Design review of the part built by this model. Coordinates are the model's own, in mm. A direction names the side the tool comes from. Round coordinates to 2 decimals unless told otherwise and drop trailing zeros. Order: outer loops, then holes, each group sorted by start corner. A loop starts at its lowest first (then second) coordinate and runs counter-clockwise, first axis right, second up.
from build123d import *

# Parameters (mm, degrees)
CROQUIS1_R              = 21.4
CROQUIS1_R_2            = 18.65
SALIENTE_EXTRUIR1_DEPTH = 26.4
CROQUIS2_R              = 18.65
SALIENTE_EXTRUIR2_DEPTH = 3
SALIENTE_EXTRUIR3_START = -4
CROQUIS3_R              = 28.5
CROQUIS3_R_2            = 21.4
SALIENTE_EXTRUIR3_DEPTH = 4
CROQUIS4_R              = 6.15
CROQUIS4_R_2            = 1.65
CORTAR_EXTRUIR1_DEPTH   = 3
CROQUIS6_R              = 2
CORTAR_EXTRUIR2_DEPTH   = 49.181531732
CROQUIS7_R              = 21.4
CROQUIS7_R_2            = 20
CORTAR_EXTRUIR3_DEPTH   = 22.4
REDONDEO1_R             = 1


with BuildPart() as part:
    # Croquis1 → Saliente-Extruir1 (new body)
    with BuildSketch(Plane.XY):
        Circle(CROQUIS1_R)
        Circle(CROQUIS1_R_2, mode=Mode.SUBTRACT)
    extrude(amount=SALIENTE_EXTRUIR1_DEPTH)

    # Croquis2 → Saliente-Extruir2 (add)
    with BuildSketch(Plane(origin=(0, 0, 0), x_dir=(-1, 0, 0), z_dir=(0, 0, -1))):
        Circle(CROQUIS2_R)
    extrude(amount=-SALIENTE_EXTRUIR2_DEPTH)

    # Croquis3 → Saliente-Extruir3 (add)
    with BuildSketch(Plane.XY.offset(26.4).offset(SALIENTE_EXTRUIR3_START)):
        Circle(CROQUIS3_R)
        Circle(CROQUIS3_R_2, mode=Mode.SUBTRACT)
    extrude(amount=SALIENTE_EXTRUIR3_DEPTH)

    # Croquis4 → Cortar-Extruir1 (cut)
    with BuildSketch(Plane(origin=(0, 0, 0), x_dir=(-1, 0, 0), z_dir=(0, 0, -1))):
        with Locations((0, -7)):
            Circle(CROQUIS4_R)
        with Locations((-15.497639275, 0.2705123)):
            Circle(CROQUIS4_R_2)
        with Locations((-7.514549114, 13.556605461)):
            Circle(CROQUIS4_R_2)
        with Locations((7.983090161, 13.286093161)):
            Circle(CROQUIS4_R_2)
        with Locations((15.497639275, -0.2705123)):
            Circle(CROQUIS4_R_2)
        with Locations((7.514549114, -13.556605461)):
            Circle(CROQUIS4_R_2)
        with Locations((-7.983090161, -13.286093161)):
            Circle(CROQUIS4_R_2)
    extrude(amount=-CORTAR_EXTRUIR1_DEPTH, mode=Mode.SUBTRACT)

    # Croquis6 → Cortar-Extruir2 (cut, through all)
    with BuildSketch(Plane.XY.offset(26.4)):
        with Locations((11.96671541, 20.688356504)):
            Circle(CROQUIS6_R)
        with Locations((23.9, -0.019301293)):
            Circle(CROQUIS6_R)
        with Locations((-11.93328459, 20.707657797)):
            Circle(CROQUIS6_R)
        with Locations((11.93328459, -20.707657797)):
            Circle(CROQUIS6_R)
        with Locations((-11.96671541, -20.688356504)):
            Circle(CROQUIS6_R)
        with Locations((-23.9, 0.019301293)):
            Circle(CROQUIS6_R)
    extrude(amount=-CORTAR_EXTRUIR2_DEPTH, mode=Mode.SUBTRACT)

    # Croquis7 → Cortar-Extruir3 (cut)
    with BuildSketch(Plane(origin=(0, 0, 0), x_dir=(-1, 0, 0), z_dir=(0, 0, -1))):
        Circle(CROQUIS7_R)
        Circle(CROQUIS7_R_2, mode=Mode.SUBTRACT)
    extrude(amount=-CORTAR_EXTRUIR3_DEPTH, mode=Mode.SUBTRACT)

    # Redondeo1
    redondeo1_edges = [part.edges().sort_by_distance(p)[0] for p in [
        (20, 0, 22.4),
    ]]
    fillet(redondeo1_edges, radius=REDONDEO1_R)


solid = part.part
1) To check wall thickness, follow line 1 along Y through (x, z) = (-0.5, 23.75); line 2 along Z through (x, y) = (-20, -12); line 3 along X through (y, z) = (-15.5, 16.25). State the ranges of each line that lie inside material, in increasing order.
Results:
line 1: y = -28.5 to -18.64, 18.64 to 28.5
line 2: z = 22.4 to 26.4
line 3: x = -12.64 to -10.37, 10.37 to 12.64
2) For faces 1 (the face through (9.97, 20.78, 24.43)), 2 (the face through (-14.8, -11.35, 14.54)), 3 (the face through (-13, -17, 22.4)), list the 3-axis set-ups (+Z, -Z, +X, -X, +Y, -Y) from which the entire face can be reached by the end or side of a thin tool; tool diameter is ignored.
Results:
face 1: +Z, -Z
face 2: +Z
face 3: -Z
3) The part is to be moulded in two halves that separate along Y. For faces 4 (the face through (-13.52, 19.49, 24.43)), 5 (the face through (6, -19, 26.4)), 6 (the face through (26.327, -10.916, 24.372)), say which applies: released by +Y, released by -Y, zero draft, split by the parting line, or undercut.
Results:
face 4: undercut
face 5: zero draft
face 6: split by the parting line
4) Clearance check with flat-ended pins moving along their axes: P1, Ø5, axis at y = 17, z = 17, coming from the +X side (3 decimals); P2, Ø4.5, axis at x = -7.98, y = 13.29, coming from the +Z side; P3, Ø12, axis at y = 13, z = 9, coming from the +X side (3 decimals); P4, Ø6.5, axis at x = -23.9, y = 0.02, coming from the +Z side. State where each tip first meets the part, or that it passes through.
Results:
P1: stops at x = 13.775
P2: stops at z = 3
P3: stops at x = 18.735
P4: stops at z = 26.4
5) Take a section at C-C on x = 7.5. State how many separate pieces and enclosed holes the cut face has, plus the area to 3 significant figures.
Results:
separate pieces: 3
enclosed holes: 0
area: 233 mm2
6) Take a section at B-B on z = 10.75. Give the boundary of the cut face in (x, y).
Results:
outline: circle Ø40 at (0, 0); hole circle Ø37.3 at (0, 0)
7) Take a section at D-D on x = 23.9. Give the boundary of the cut face in (y, z), plus the area to 3 significant figures.
Results:
outline: (-15.53, 22.4) - (-2.02, 22.4) - (-2.02, 26.4) - (-15.53, 26.4) - close; (1.98, 22.4) - (15.53, 22.4) - (15.53, 26.4) - (1.98, 26.4) - close
area: 108 mm2
8) Take a section at A-A on x = 0. Give the boundary of the cut face in (y, z), plus the area to 3 significant figures.
Results:
outline: (-28.5, 22.4) - (-21, 22.4) arc R1 cw to (-20, 21.4) - (-20, 0) - (-13.15, 0) - (-13.15, 3) - (-18.65, 3) - (-18.65, 26.4) - (-28.5, 26.4) - close; (-0.85, 0) - (20, 0) - (20, 21.4) arc R1 cw to (21, 22.4) - (28.5, 22.4) - (28.5, 26.4) - (18.65, 26.4) - (18.65, 3) - (-0.85, 3) - close
area: 215 mm2
